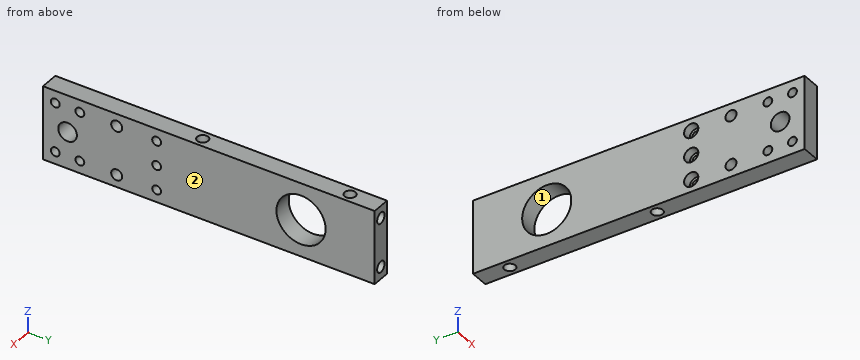
from build123d import *

# Parameters (mm, degrees)
SKETCH_W        = 171.45
SKETCH_H        = 38.1
SKETCH_R        = 4.826
SKETCH_R_2      = 2.286
SKETCH_R_3      = 12.7
SKETCH_R_4      = 2.8575
PAD_DEPTH       = 9.525
SKETCH001_R     = 2.8575
POCKET_DEPTH    = 6.096
SKETCH086_R     = 2.8575
POCKET014_DEPTH = 6.096
SKETCH087_R     = 2.8575
POCKET015_DEPTH = 6.096
SKETCH094_R     = 3.683
POCKET022_DEPTH = 4.318


with BuildPart() as left_wall:
    # Sketch → Pad (new body)
    with BuildSketch(Plane.YZ):
        Rectangle(SKETCH_W, SKETCH_H)
        with Locations((-73.025, 0)):
            Circle(SKETCH_R, mode=Mode.SUBTRACT)
        with Locations((-26.9875, 12.7)):
            Circle(SKETCH_R_2, mode=Mode.SUBTRACT)
        with Locations((-26.9875, -12.7)):
            Circle(SKETCH_R_2, mode=Mode.SUBTRACT)
        with Locations((47.625, 0)):
            Circle(SKETCH_R_3, mode=Mode.SUBTRACT)
        with Locations((-79.375, -12.7)):
            Circle(SKETCH_R_2, mode=Mode.SUBTRACT)
        with Locations((-66.675, -12.7)):
            Circle(SKETCH_R_2, mode=Mode.SUBTRACT)
        with Locations((-47.625, 12.7)):
            Circle(SKETCH_R_4, mode=Mode.SUBTRACT)
        with Locations((-47.625, -12.7)):
            Circle(SKETCH_R_4, mode=Mode.SUBTRACT)
        with Locations((-26.9875, 0)):
            Circle(SKETCH_R_2, mode=Mode.SUBTRACT)
        with Locations((-79.375, 12.7)):
            Circle(SKETCH_R_2, mode=Mode.SUBTRACT)
        with Locations((-66.675, 12.7)):
            Circle(SKETCH_R_2, mode=Mode.SUBTRACT)
    extrude(amount=PAD_DEPTH)

    # Sketch001 (on Face3 of Pad) → Pocket (cut)
    with BuildSketch(Plane.ZX.offset(85.725)):
        with Locations((12.7, 4.74788)):
            Circle(SKETCH001_R)
        with Locations((-12.7, 4.74788)):
            Circle(SKETCH001_R)
    extrude(amount=-POCKET_DEPTH, mode=Mode.SUBTRACT)

    # Sketch086 (on Face2 of Pocket) → Pocket014 (cut)
    with BuildSketch(Plane(origin=(0, 0, 19.05), x_dir=(0, -1, 0), z_dir=(0, 0, 1))):
        with Locations((-69.85, 4.7625)):
            Circle(SKETCH086_R)
        with Locations((6.35, 4.7625)):
            Circle(SKETCH086_R)
    extrude(amount=-POCKET014_DEPTH, mode=Mode.SUBTRACT)

    # Sketch087 (on Face3 of Pocket) → Pocket015 (cut)
    with BuildSketch(Plane.YX.offset(19.05)):
        with Locations((-6.35, 4.7625)):
            Circle(SKETCH087_R)
        with Locations((69.85, 4.7625)):
            Circle(SKETCH087_R)
    extrude(amount=-POCKET015_DEPTH, mode=Mode.SUBTRACT)

    # Sketch094 (on Face5 of Pocket015) → Pocket022 (cut)
    with BuildSketch(Plane.YZ.offset(9.525)):
        with Locations((-27.051, 12.7)):
            Circle(SKETCH094_R)
        with Locations((-27.051, -12.7)):
            Circle(SKETCH094_R)
        with Locations((-27.051, 0)):
            Circle(SKETCH094_R)
    extrude(amount=-POCKET022_DEPTH, mode=Mode.SUBTRACT)


with BuildPart() as left_wall_1:
    # Body placement: moved
    add(left_wall.part.moved(Location((0, 3.556, 0))))


with BuildPart() as right_wall:
    # Part__Mirroring: instance of left-wall
    add(left_wall_1.part.mirror(Plane(origin=(0, 0, 0), x_dir=(0, -1, 0), z_dir=(1, 0, 0))))


with BuildPart() as right_wall_1:
    # Part__Mirroring placement: moved
    add(right_wall.part.moved(Location((-134.112, 0, 0))))


solid = right_wall_1.part
The listing builds one solid part. Answer for the finished solid, in the listing's coordinates (mm). Face numbers are marked on the shaded views. Give positions to 0.01 mm unless a question says otherwise; leave off trailing zeros. Loops run counter-clockwise (first coordinate to the right, second up) from the corner with the lowest first, then second, coordinate; pieces in that order, holes last. Notation, with made-up numbers: M -35,19 L -19,19 A25 cw -19,56 Z; hole C -15.75,0.5 d4. An arc over 180 degrees is marked long. Answer as CSV lines item,"result".
Item 1: Given pin 1 Ø8.5 at (y, z) = (-23.495, 0) entering from -X; pin 2 Ø3.5 at (x, y) = (-138.87, 73.41) entering from -Z; pin 3 Ø3 at (x, z) = (-138, 13.5) entering from +Y (3 decimals); pin 4 Ø2 at (y, z) = (-24, -12) entering from -X, each flat-ended and moving along its own axis, determine where each tip first touches the part or whether it passes through.
Values follow:
pin 1,"stops at x = -143.64"
pin 2,"stops at z = -12.95"
pin 3,"stops at y = 83.185"
pin 4,"passes through"
Item 2: The part is cut by section A-A (z = 0). Give the vertices of the cut face in (x, y) (1 decimal), and give its area (3 significant figures).
Values follow:
outline,"M -143.6,-82.2 L -134.1,-82.2 L -134.1,-74.3 L -143.6,-74.3 Z; M -143.6,-64.6 L -134.1,-64.6 L -134.1,-25.7 L -139.3,-25.7 L -139.3,-27.2 L -143.6,-27.2 Z; M -143.6,-19.8 L -139.3,-19.8 L -139.3,-21.1 L -134.1,-21.1 L -134.1,38.5 L -143.6,38.5 Z; M -143.6,63.9 L -134.1,63.9 L -134.1,89.3 L -143.6,89.3 Z"
area,"1,240 mm^2"
Item 3: Straight lines are drawn through the part: line 1 along Y through (x, z) = (-139, -17); line 2 along Z through (x, y) = (-134.75, 50.5); line 3 along Z through (x, y) = (-136.75, -23). For each, find the intervals that lie inside material, in ascending order. Write a range as [from, to].
Values follow:
line 1,"y = [-82.17, -5.65], [0.06, 70.55], [76.26, 89.28]"
line 2,"z = [-19.05, -12.68], [12.68, 19.05]"
line 3,"z = [-19.05, -14.94], [-10.46, -2.24], [2.24, 10.46], [14.94, 19.05]"
Item 4: The part is cut by section B-B (y = 41.5). Give the vertices of the cut face in (x, z).
Values follow:
outline,"M -143.64,-19.05 L -134.11,-19.05 L -134.11,-8.22 L -143.64,-8.22 Z; M -143.64,8.22 L -134.11,8.22 L -134.11,19.05 L -143.64,19.05 Z"
Item 5: The mould has two halves that part along Y. Classify the marked faces 1 and 2: released by +Y, released by -Y, zero draft, split by the parting line, or undercut.
Values follow:
face 1,"undercut"
face 2,"zero draft"
